```python
from build123d import *

# Parameters (mm, degrees)
SALIENTE_EXTRUIR1_DEPTH     = 100
CORTAR_EXTRUIR2_DEPTH       = 26
CORTAR_EXTRUIR2_DEPTH_BACK  = 26
CROQUIS3_R                  = 13.5
CROQUIS11_W                 = 7.2
CROQUIS11_H                 = 7.2
CORTAR_EXTRUIR6_DEPTH       = 6
CROQUIS12_W                 = 5.5
CROQUIS12_H                 = 5.5
CORTAR_EXTRUIR7_DEPTH       = 6
CORTAR_EXTRUIR11_DEPTH      = 110.476024773
CORTAR_EXTRUIR11_DEPTH_BACK = 110.476024773
SALIENTE_EXTRUIR2_DEPTH     = 100


with BuildPart() as part:
    # Croquis1 → Saliente-Extruir1 (new body)
    with BuildSketch(Plane.XY):
        with BuildLine():
            Line((0, 0), (11, 0))
            Line((11, 0), (11, 4))
            Line((11, 4), (44, 7))
            Line((44, 7), (44, 4))
            ThreePointArc((44, 4), (39.101020514, 1.464101615), (38.343145751, -4))
            Line((38.343145751, -4), (0, -4))
            Line((0, -4), (0, 0))
        make_face()
    extrude(amount=SALIENTE_EXTRUIR1_DEPTH)

    # Croquis3 → Cortar-Extruir2 (cut, two sides: drawn at the far end of the back side and taken through both)
    with BuildSketch(Plane.XY.offset(50).offset(-CORTAR_EXTRUIR2_DEPTH_BACK)):
        with Locations((44, -2)):
            Circle(CROQUIS3_R)
    extrude(amount=CORTAR_EXTRUIR2_DEPTH + CORTAR_EXTRUIR2_DEPTH_BACK, mode=Mode.SUBTRACT)

    # Croquis11 → Cortar-Extruir6 (cut)
    with BuildSketch(Plane(origin=(-0.270491803, 2.975409836, 0), x_dir=(0.995893206467704, 0.09053574604251857, 0), z_dir=(-0.09053574604251857, 0.995893206467704, 0))):
        with Locations((26.442986434, -50)):
            Rectangle(CROQUIS11_W, CROQUIS11_H)
    extrude(amount=-CORTAR_EXTRUIR6_DEPTH, mode=Mode.SUBTRACT)

    # Croquis12 → Cortar-Extruir7 (cut)
    with BuildSketch(Plane(origin=(0.272722673, -2.999949403, 0), x_dir=(0.995893206467704, 0.09053574604251854, 0), z_dir=(-0.09053574604251854, 0.995893206467704, 0))):
        with Locations((26.442986434, -50)):
            Rectangle(CROQUIS12_W, CROQUIS12_H)
    extrude(amount=-CORTAR_EXTRUIR7_DEPTH, mode=Mode.SUBTRACT)

    # Croquis14 → Cortar-Extruir11 (cut, two sides: drawn at the far end of the back side and taken through both)
    with BuildSketch(Plane.XY.offset(100).offset(-CORTAR_EXTRUIR11_DEPTH_BACK)):
        with BuildLine():
            Line((33.134740511, -104.708323764), (33.134740511, -4))
            ThreePointArc((33.134740511, -4), (36.309024056, 3.730683407), (44, 7))
            Line((44, 7), (144.700675445, 8.241144726))
            Line((144.700675445, 8.241144726), (287.998687156, -133.301589954))
            Line((287.998687156, -133.301589954), (176.432752222, -246.251058444))
            Line((176.432752222, -246.251058444), (33.134740511, -104.708323764))
        make_face()
    extrude(amount=CORTAR_EXTRUIR11_DEPTH + CORTAR_EXTRUIR11_DEPTH_BACK, mode=Mode.SUBTRACT)

    # Croquis15 → Saliente-Extruir2 (add)
    with BuildSketch(Plane.XY.offset(100)):
        with BuildLine():
            Line((0, -4), (0, -15))
            ThreePointArc((0, -15), (3.001359468, -8.695211228), (8.169871019, -4))
            Line((8.169871019, -4), (0, -4))
        make_face()
    extrude(amount=-SALIENTE_EXTRUIR2_DEPTH)


solid = part.part
```
Check sheet for the modelled part. Datum: model origin and axes. Units: mm. A direction names the side the tool comes from. Round coordinates to 2 decimals unless told otherwise and drop trailing zeros. Write each loop counter-clockwise with the first axis right and the second up, starting at its lowest first coordinate (ties: lowest second). Pieces come first, ordered by that corner, then holes. Notation, with made-up numbers: (10, 85.5) -> (67, 85.5) arc R32 cw to (67, 124.5) -> close; hole circle Ø1 at (25, -37.5). An arc over 180 degrees is marked (long way). Put each result on its own line as item: value.
(1) Sectioned sample at C-C (z = 17.5). Enter the section's corners in (x, y).
Values found:
outline: (0, -15) arc R18.06 cw to (8.17, -4) -> (33.13, -4) arc R11 cw to (42.29, 6.84) -> (11, 4) -> (11, 0) -> (0, 0) -> close
(2) Mould release check, pull along Z, two halves, no side actions. Record for faces 6 (the face through (18, 0, 0)), 7 (the face through (26, 2, 53.6)), 8 (the face through (21, -4, 49)): released by +Z, released by -Z, zero draft, split by the parting line, or undercut.
Values found:
face 6: released by -Z
face 7: undercut
face 8: zero draft
(3) Material ranges on line 1 (Y direction, x = 12, z = 58.5); line 2 (X direction, y = -10, z = 9); line 3 (Y direction, x = 9, z = 31), recorded low to high.
Values found:
line 1: y = -4 to 4.09
line 2: x = 0 to 2.12
line 3: y = -4 to 0
(4) Sectioned sample at B-B (y = 2.5). Enter the section's corners in (x, z).
Values found:
outline: (11, 0) -> (35.26, 0) -> (35.26, 24) -> (31.27, 24) -> (31.27, 76) -> (35.26, 76) -> (35.26, 100) -> (11, 100) -> close; hole (22.71, 46.4) -> (29.94, 46.4) -> (29.94, 53.6) -> (22.71, 53.6) -> close
(5) Tool access check on faces 1 (the face through (2.943, -8.774, 50.7)), 2 (the face through (22.746, 2.098, 50.05)), 3 (the face through (30.916, 1.325, 49.636)), 4 (the face through (5, 0, 49)), 5 (the face through (29.51, -2.15, 50.04)). Record the directions out of +Z, -Z, +X, -X, +Y, -Y that give a thin tool (end or side, any length) a straight path to the whole face; none if there is none.
Values found:
face 1: +Z, -Z, +X, -Y
face 2: +Y
face 3: +X
face 4: +Z, -Z, -X, +Y
face 5: -Y
(6) Go/stop test with flat-tipped pins: pin 1 Ø10 at (x, z) = (6.5, 20.5) entering from -Y; pin 2 Ø5 at (y, z) = (-12.5, 66.5) entering from +X; pin 3 Ø10 at (x, z) = (17.5, 53) entering from +Y; pin 4 Ø3.5 at (x, y) = (36, 0) entering from +Z. Record where each tip stops, or that it passes through.
Values found:
pin 1: stops at y = -11.09
pin 2: stops at x = 2.12
pin 3: stops at y = 5.04
pin 4: passes through
(7) Sectioned sample at D-D (z = 50). Enter the section's corners in (x, y).
Values found:
outline: (0, -15) arc R18.06 cw to (8.17, -4) -> (24.15, -4) -> (23.87, -0.85) -> (23.02, -0.93) -> (22.48, 5.04) -> (11, 4) -> (11, 0) -> (0, 0) -> close; (29.35, -0.36) -> (29.68, -4) -> (30.65, -4) arc R13.5 cw to (33.13, 6.01) -> (29.65, 5.7) -> (30.19, -0.28) -> close
(8) Sectioned sample at A-A (x = 28). Enter the section's corners in (y, z).
Values found:
outline: (-4, 0) -> (5.55, 0) -> (5.55, 46.4) -> (-0.48, 46.4) -> (-0.48, 47.25) -> (-4, 47.25) -> close; (-4, 52.75) -> (-0.48, 52.75) -> (-0.48, 53.6) -> (5.55, 53.6) -> (5.55, 100) -> (-4, 100) -> close
